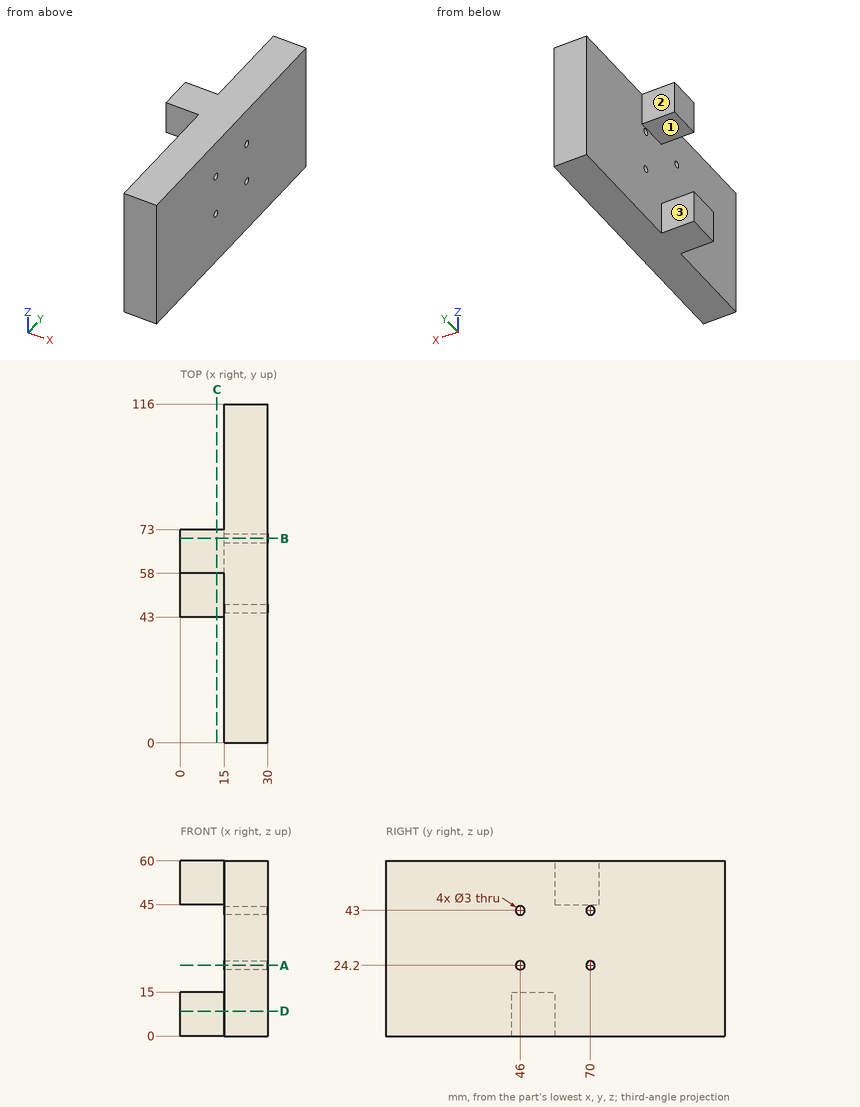
Source: three-view drawing plus pictorial views. Frame: mm from the lowest corner of the part. A direction names the side the tool comes from. Give positions to 0.01 mm unless a question says otherwise; leave off trailing zeros. Loops run counter-clockwise (first coordinate to the right, second up) from the corner with the lowest first, then second, coordinate; pieces in that order, holes last. Notation, with made-up numbers: (69.25, 49) -> (120.25, 49) arc R24 ccw to (120.25, 71) -> close; hole circle Ø7 at (1.25, 12). An arc over 180 degrees is marked (long way). Use a Markdown table: item, result. Add a question column.
(1) Section query C-C (x = 12.5). Output: boundary loops of the cut face in (y, z).
(2) Ray query, line 1 (Z direction, x = 20.25, y = 70); line 2 (Y direction, x = 24.25, z = 24.2); line 3 (X direction, y = 76, z = 24). Return the intervals inside material, ascending.
(3) Section query A-A (z = 24.2). Output: boundary loops of the cut face in (x, y), then the cut area to 3 significant figures.
(4) Access query for the marked faces 1, 2 and 3. Directions: +Z, -Z, +X, -X, +Y, -Y. A direction counts if a zero-diameter tool reaches every point of the face in a straight line with its end or side. Return the directions, or none.
(5) First-contact query: pin 1 Ø4 at (y, z) = (70, 24.2) entering from +X; pin 2 Ø7.5 at (x, y) = (7, 52.5) entering from +Z; pin 3 Ø1.8 at (y, z) = (70, 43) entering from -X; pin 4 Ø12 at (x, z) = (5.5, 50.5) entering from -Y. Flat tips, straight axial feed; report the tip coordinate or a pass-through.
(6) Section query D-D (z = 8.5). Output: boundary loops of the cut face in (x, y).
(7) Section query B-B (y = 70). Output: boundary loops of the cut face in (x, z).
Checked values:
| question | item | result |
|---|---|---|
| 1 | outline | (43, 0) -> (58, 0) -> (58, 15) -> (43, 15) -> close; (58, 45) -> (73, 45) -> (73, 60) -> (58, 60) -> close |
| 2 | line 1 | 0 to 22.7, 25.7 to 41.5, 44.5 to 60 |
| 2 | line 2 | 0 to 44.5, 47.5 to 68.5, 71.5 to 116 |
| 2 | line 3 | 15 to 30 |
| 3 | outline | (15, 0) -> (30, 0) -> (30, 44.5) -> (15, 44.5) -> close; (15, 47.5) -> (30, 47.5) -> (30, 68.5) -> (15, 68.5) -> close; (15, 71.5) -> (30, 71.5) -> (30, 116) -> (15, 116) -> close |
| 3 | area | 1,650 mm^2 |
| 4 | face 1 | -Z, -X, +Y, -Y |
| 4 | face 2 | +Z, -Z, -X, +Y |
| 4 | face 3 | -Z, -X, +Y |
| 5 | pin 1 | x = 30 |
| 5 | pin 2 | z = 15 |
| 5 | pin 3 | through |
| 5 | pin 4 | y = 58 |
| 6 | outline | (0, 43) -> (15, 43) -> (15, 0) -> (30, 0) -> (30, 116) -> (15, 116) -> (15, 58) -> (0, 58) -> close |
| 7 | outline | (0, 45) -> (15, 45) -> (15, 44.5) -> (30, 44.5) -> (30, 60) -> (0, 60) -> close; (15, 0) -> (30, 0) -> (30, 22.7) -> (15, 22.7) -> close; (15, 25.7) -> (30, 25.7) -> (30, 41.5) -> (15, 41.5) -> close |
